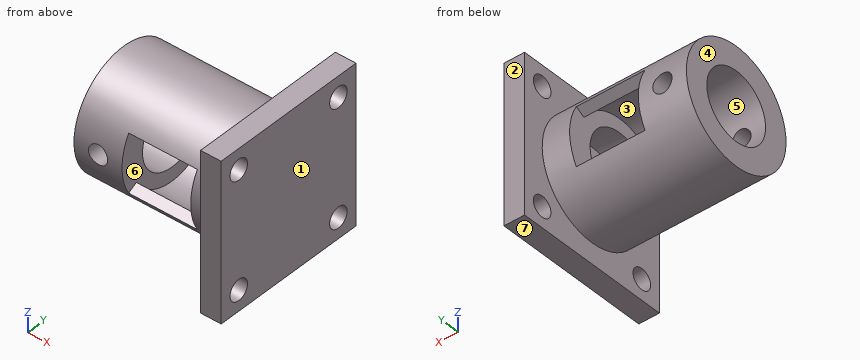
from build123d import *

# Parameters (mm, degrees)
SKETCH012_R             = 8.5
SKETCH012_R_2           = 5.0125
PAD009_DEPTH            = 21
SKETCH013_W             = 2
SKETCH013_H             = 10
SKETCH014_W             = 1.4875
SKETCH014_H             = 10
GROOVE002_ANGLE         = -60
SKETCH015_R             = 1.4
POCKET002_DEPTH         = 8.501
POCKET002_DEPTH_BACK    = 8.501
SKETCH016_W             = 23
SKETCH016_H             = 23
SKETCH016_R             = 1.5
PAD010_DEPTH            = 3
BODY006_PLACEMENT_ANGLE = 90


with BuildPart() as part:
    # Sketch012 → Pad009 (new body)
    with BuildSketch(Plane.XY):
        Circle(SKETCH012_R)
        Circle(SKETCH012_R_2, mode=Mode.SUBTRACT)
    extrude(amount=PAD009_DEPTH)

    # Sketch013 → Groove001 (revolve, cut)
    with BuildSketch(Plane.YZ):
        with Locations((-6.0125, 12)):
            Rectangle(SKETCH013_W, SKETCH013_H)
        with Locations((6.0125, 12)):
            Rectangle(SKETCH013_W, SKETCH013_H)
    revolve(axis=Axis((0, 0, 0), (0, 0, 1)), mode=Mode.SUBTRACT)

    # Sketch014 → Groove002 (revolve, symmetric, cut)
    with BuildSketch(Plane.YZ) as groove002_sk:
        with Locations((-7.75625, 12)):
            Rectangle(SKETCH014_W, SKETCH014_H)
        with Locations((7.75625, 12)):
            Rectangle(SKETCH014_W, SKETCH014_H)
    revolve(axis=Axis((0, 0, 0), (0, 0, 1)), revolution_arc=GROOVE002_ANGLE / 2, mode=Mode.SUBTRACT)
    revolve(groove002_sk.sketch, axis=Axis((0, 0, 0), (0, 0, -1)), revolution_arc=GROOVE002_ANGLE / 2, mode=Mode.SUBTRACT)

    # Sketch015 → Pocket002 (cut, two sides)
    with BuildSketch(Plane.XZ) as pocket002_sk:
        with Locations((0, 3.5)):
            Circle(SKETCH015_R)
    extrude(amount=-POCKET002_DEPTH, mode=Mode.SUBTRACT)
    extrude(pocket002_sk.sketch, amount=POCKET002_DEPTH_BACK, mode=Mode.SUBTRACT)

    # Sketch016 → Pad010 (join)
    with BuildSketch(Plane.XY.offset(21)):
        Rectangle(SKETCH016_W, SKETCH016_H)
        with Locations((-8.5, 8.5)):
            Circle(SKETCH016_R, mode=Mode.SUBTRACT)
        with Locations((-8.5, -8.5)):
            Circle(SKETCH016_R, mode=Mode.SUBTRACT)
        with Locations((8.5, 8.5)):
            Circle(SKETCH016_R, mode=Mode.SUBTRACT)
        with Locations((8.5, -8.5)):
            Circle(SKETCH016_R, mode=Mode.SUBTRACT)
    extrude(amount=PAD010_DEPTH)


with BuildPart() as part_1:
    # Body006 placement: moved
    add(part.part.moved(Location((-27, 13.5, 11.5))).rotate(Axis((-27, 13.5, 11.5), (0, 1, 0)), BODY006_PLACEMENT_ANGLE))


solid = part_1.part
Read the model definition and answer for the solid it produces. Units are mm, in the model's axes. Face numbers are marked on the shaded views. A direction names the side the tool comes from. Round coordinates to 2 decimals unless told otherwise and drop trailing zeros. Order: outer loops, then holes, each group sorted by start corner. A loop starts at its lowest first (then second) coordinate and runs counter-clockwise, first axis right, second up. Notation, with made-up numbers: (62, 38) - (84, 38) arc R19 cw to (84, 58) - close; hole circle Ø3 at (-33, 71). An arc over 180 degrees is marked (long way). Use one line per item in the form item = value. Start each with the question number.
(1) The part is cut by section C-C (y = 13.5). Give the vertices of the cut face in (x, z).
(2) Determine the mould class of the marked faces 1, 2, 3 and 4 for opening direction X: +X half, -X half, draft (parallel to the pull), parting line (faces both ways), or undercut.
(3) The part is cut by section B-B (z = 11.5). Give the vertices of the cut face in (x, y).
(4) The part is cut by section D-D (z = 8.5). Give the vertices of the cut face in (x, y), then the cut area to 3 significant figures.
(5) Find the intervals of material crossed by line 1 along X through (y, z) = (6.3, 11.5); line 2 along Y through (x, z) = (-4.2, 3); line 3 along X through (y, z) = (18, 16), in increasing order. Write a range as from..to.
(6) Flat-ended cylindrical pins translate along their axes: pin 1 Ø5 at (x, y) = (-11, 7) entering from +Z; pin 2 Ø1.7 at (x, z) = (-23.5, 11.5) entering from -Y; pin 3 Ø4 at (x, y) = (-19.5, 20.5) entering from -Z; pin 4 Ø5 at (x, z) = (-18.5, 7) entering from -Y. Find the tip coordinate at first contact, or state that the pin passes through.
(7) For the marked faces 5, 6 and 7, determine the directions among +Z, -Z, +X, -X, +Y, -Y from which every point of the face is accessible in a straight line to the end or side of a thin tool.
Checked values:
q1.outline = (-27, 3) - (-6, 3) - (-6, 0) - (-3, 0) - (-3, 23) - (-6, 23) - (-6, 20) - (-27, 20) - (-27, 16.51) - (-20, 16.51) - (-20, 18.51) - (-10, 18.51) - (-10, 16.51) - (-6, 16.51) - (-6, 6.49) - (-10, 6.49) - (-10, 4.49) - (-20, 4.49) - (-20, 6.49) - (-27, 6.49) - close
q2.face_1 = +X half
q2.face_2 = draft
q2.face_3 = undercut
q2.face_4 = -X half
q3.outline = (-27, 5) - (-24.9, 5) - (-24.9, 8.49) - (-27, 8.49) - close; (-27, 18.51) - (-24.9, 18.51) - (-24.9, 22) - (-27, 22) - close; (-22.1, 5) - (-20, 5) - (-20, 8.49) - (-22.1, 8.49) - close; (-22.1, 18.51) - (-20, 18.51) - (-20, 22) - (-22.1, 22) - close; (-10, 5) - (-6, 5) - (-6, 2) - (-3, 2) - (-3, 25) - (-6, 25) - (-6, 22) - (-10, 22) - (-10, 18.51) - (-6, 18.51) - (-6, 8.49) - (-10, 8.49) - close
q4.outline = (-27, 5.55) - (-20, 5.55) - (-20, 9.48) - (-27, 9.48) - close; (-27, 17.52) - (-20, 17.52) - (-20, 21.45) - (-27, 21.45) - close; (-10, 5.55) - (-6, 5.55) - (-6, 2) - (-3, 2) - (-3, 25) - (-6, 25) - (-6, 21.45) - (-10, 21.45) - (-10, 17.52) - (-6, 17.52) - (-6, 9.48) - (-10, 9.48) - close
q4.area = 156 mm^2
q5.line_1 = -27..-24.9, -22.1..-20, -10..-3
q5.line_2 = 2..3.5, 6.5..20.5, 23.5..25
q5.line_3 = -27..-20, -10..-3
q6.pin_1 = 19
q6.pin_2 = through
q6.pin_3 = 4.63
q6.pin_4 = 5.38
q7.face_5 = -X
q7.face_6 = none
q7.face_7 = -Z, +X, -X, +Y, -Y
